CAD build for the part. Positions are in the model's coordinates, mm. Give positions to 0.01 mm unless a question says otherwise; leave off trailing zeros. Loops run counter-clockwise (first coordinate to the right, second up) from the corner with the lowest first, then second, coordinate; pieces in that order, holes last. Notation, with made-up numbers: M -33.5,7 L 8.5,7 A10 ccw 8.5,25 Z; hole C 65.5,35.5 d9. An arc over 180 degrees is marked long. Answer as CSV lines item,"result".
```python
from build123d import *

# Parameters (mm, degrees)
SKETCH_1_R      = 5.05
SKETCH_1_R_2    = 2.05
SKETCH_1_R_3    = 4
EXTRUDE_1_DEPTH = 2


with BuildPart() as part:
    # 草图1 → 凸台-拉伸1 (new body)
    with BuildSketch(Plane.XY):
        with BuildLine():
            Line((-2.587732913, 20.736278596), (-2.587732913, 27.736278596))
            Line((-2.587732913, 27.736278596), (1.262267087, 27.736278596))
            Line((1.262267087, 27.736278596), (1.262267087, 33.336278596))
            Line((1.262267087, 33.336278596), (-2.687732913, 33.336278596))
            Line((-2.687732913, 33.336278596), (-12.587732913, 33.336278596))
            Line((-12.587732913, 33.336278596), (-16.537732913, 33.336278596))
            Line((-16.537732913, 33.336278596), (-16.537732913, 27.736278596))
            Line((-16.537732913, 27.736278596), (-12.687732913, 27.736278596))
            Line((-12.687732913, 27.736278596), (-12.687732913, 20.736278596))
            Line((-12.687732913, 20.736278596), (-18.637732913, 20.736278596))
            Line((-18.637732913, 20.736278596), (-18.637732913, 14.736278596))
            Line((-18.637732913, 14.736278596), (-26.637732913, 14.736278596))
            Line((-26.637732913, 14.736278596), (-26.637732913, 20.736278596))
            Line((-26.637732913, 20.736278596), (-30.637732913, 20.736278596))
            Line((-30.637732913, 20.736278596), (-30.637732913, 51.623197149))
            ThreePointArc((-30.637732913, 51.623197149), (-7.637732913, 123.236278596), (15.362267087, 51.623197149))
            Line((15.362267087, 51.623197149), (15.362267087, 20.736278596))
            Line((15.362267087, 20.736278596), (11.362267087, 20.736278596))
            Line((11.362267087, 20.736278596), (11.362267087, 14.736278596))
            Line((11.362267087, 14.736278596), (3.362267087, 14.736278596))
            Line((3.362267087, 14.736278596), (3.362267087, 20.736278596))
            Line((3.362267087, 20.736278596), (-2.587732913, 20.736278596))
        make_face()
        with Locations((-7.637732913, 83.736278596)):
            Circle(SKETCH_1_R, mode=Mode.SUBTRACT)
        with Locations((10.039936617, 66.058609066)):
            Circle(SKETCH_1_R_2, mode=Mode.SUBTRACT)
        with Locations((-25.315402443, 66.058609066)):
            Circle(SKETCH_1_R_2, mode=Mode.SUBTRACT)
        with Locations((-25.315402443, 101.413948126)):
            Circle(SKETCH_1_R_2, mode=Mode.SUBTRACT)
        with Locations((10.039936617, 101.413948126)):
            Circle(SKETCH_1_R_2, mode=Mode.SUBTRACT)
        with Locations((-7.637732913, 48.536278596)):
            Circle(SKETCH_1_R_3, mode=Mode.SUBTRACT)
    extrude(amount=EXTRUDE_1_DEPTH)


solid = part.part
```
Q1. Cut at B-B (x = 9.5). Write the cut outline in (y, z).
Solution:
outline,"M 14.74,0 L 64.08,0 L 64.08,2 L 14.74,2 Z; M 68.04,0 L 99.44,0 L 99.44,2 L 68.04,2 Z; M 103.39,0 L 119.32,0 L 119.32,2 L 103.39,2 Z"
Q2. Wall check: line 1 (X direction, y = 21, z = 1.05); line 2 (X direction, y = 30, z = 1.4); line 3 (Y direction, x = -27, z = 0.5). Give the ranges that are in metal, low to high. Write a range as [from, to].
Solution:
line 1,"x = [-30.64, -12.69], [-2.59, 15.36]"
line 2,"x = [-30.64, -16.54], [1.26, 15.36]"
line 3,"y = [20.74, 64.89], [67.23, 100.25], [102.58, 118.17]"
Q3. Cut at A-A (y = 87.5). Write the cut outline in (x, z).
Solution:
outline,"M -46.96,0 L -11,0 L -11,2 L -46.96,2 Z; M -4.27,0 L 31.68,0 L 31.68,2 L -4.27,2 Z"
Q4. Cut at C-C (z = 1.4). Write the cut outline in (x, y).
Solution:
outline,"M -30.64,20.74 L -26.64,20.74 L -26.64,14.74 L -18.64,14.74 L -18.64,20.74 L -12.69,20.74 L -12.69,27.74 L -16.54,27.74 L -16.54,33.34 L 1.26,33.34 L 1.26,27.74 L -2.59,27.74 L -2.59,20.74 L 3.36,20.74 L 3.36,14.74 L 11.36,14.74 L 11.36,20.74 L 15.36,20.74 L 15.36,51.62 A39.5 ccw long -30.64,51.62 Z; hole C -25.32,66.06 d4.1; hole C -25.32,101.41 d4.1; hole C -7.64,83.74 d10.1; hole C -7.64,48.54 d8; hole C 10.04,66.06 d4.1; hole C 10.04,101.41 d4.1"
Q5. Cut at D-D (y = 47). Write the cut outline in (x, z).
Solution:
outline,"M -30.64,0 L -11.33,0 L -11.33,2 L -30.64,2 Z; M -3.94,0 L 15.36,0 L 15.36,2 L -3.94,2 Z"
Q6. Mould opens along Y. For faces 1 (the cylindrical face through (-26.94, 64.81, 0.99)), 2 (the cylindrical face through (-9.03, 123.21, 0.99)), 3 (the flat face through (-7, 70, 0)) say: released by +Y, released by -Y, zero draft, split by the parting line, or undercut.
Solution:
face 1,"undercut"
face 2,"split by the parting line"
face 3,"zero draft"
Q7. Pin check, flat tips, straight feed: P1, Ø1, axis at y = 30, z = 1, coming from the +X side; P2, Ø1, axis at x = 13, z = 1.5, coming from the -Y side; P3, Ø5.5, axis at x = 10.04, y = 101.41, coming from the -Z side; P4, Ø0.6, axis at x = -13.5, z = 1, coming from the +Y side. Stop position of each tip, or through.
Solution:
P1,"stops at x = 15.36"
P2,"stops at y = 20.74"
P3,"stops at z = 0"
P4,"stops at y = 122.84"
